Geometry check sheet. Reference: the model listing, model coordinates, mm. Face numbers are marked on the shaded views. Round coordinates to 2 decimals unless told otherwise and drop trailing zeros. Loops run counter-clockwise (first coordinate to the right, second up) from the corner with the lowest first, then second, coordinate; pieces in that order, holes last. Notation, with made-up numbers: M -10,82.5 L 5,82.5 A29 cw 5,113.5 Z; hole C 72.5,-19.75 d4. An arc over 180 degrees is marked long. Answer in a Markdown table with one row per item. Add a question column.
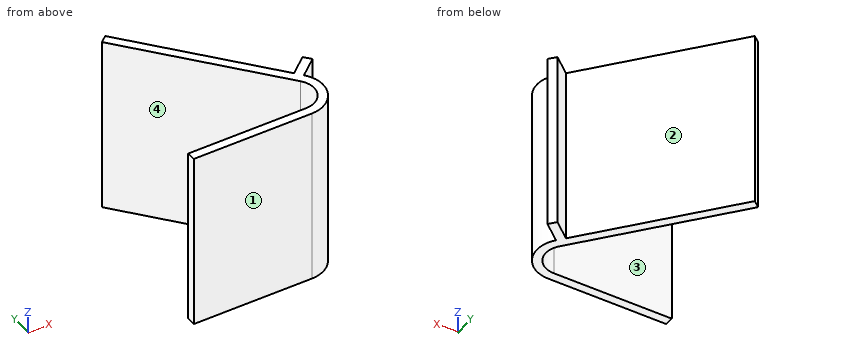
```python
from build123d import *

# Parameters (mm, degrees)
F1_DEPTH = 152.4


with BuildPart() as f1:
    # F0 (on Top) → F1 (new body)
    with BuildSketch(Plane.XY):
        with BuildLine():
            Line((-114.31821, -32.882527), (-114.198142, -40.501581))
            Line((-114.198142, -40.501581), (-12.598142, -40.501581))
            ThreePointArc((-12.598142, -40.501581), (10.422075, -25.836085), (6.859386, 1.225224))
            Line((6.859386, 1.225224), (22.425409, 14.286668))
            Line((22.425409, 14.286668), (17.527368, 20.123927))
            Line((17.527368, 20.123927), (1.961345, 7.062483))
            Line((1.961345, 7.062483), (-91.101445, 117.970397))
            Line((-91.101445, 117.970397), (-96.938704, 113.072356))
            Line((-96.938704, 113.072356), (1.022921, -3.673763))
            ThreePointArc((1.022921, -3.673763), (3.516804, -22.61668), (-12.597349, -32.882527))
            Line((-12.597349, -32.882527), (-114.31821, -32.882527))
        make_face()
    extrude(amount=F1_DEPTH)


solid = f1.part
```
1) Cross-section at A-A, the plane z = 85. Record the boundary of the cut face in (x, y), plus the area to 3 significant figures.
2) Cross-section at C-C, the plane x = -100.5. Record the boundary of the cut face in (y, z).
3) Thickness scan on L1, parallel to Y at x = -106, z = 68.5; L2, parallel to Y at x = -76, z = 143; L3, parallel to X at y = 14, z = 54.5. Record the ranges inside material, lowest first. Write a range as [from, to].
4) Cross-section at D-D, the plane y = 106. Record the boundary of the cut face in (x, z).
5) Go/stop test with flat-tipped pins: pin 1 (10 mm diameter, centred on x = -95.5, z = 124, fed in from +Y); pin 2 (6 mm diameter, centred on y = 18.5, z = 38.5, fed in from -X); pin 3 (12 mm diameter, centred on x = -4.5, z = 84, fed in from +Y). Record where each tip stops, or that it passes through.
6) Draft check along Y on the marked faces 1, 2, 3 and 4. Enter one of: +Y half, -Y half, draft (parallel to the pull), parting line (faces both ways), or undercut.
7) Cross-section at B-B, the plane x = -18. Record the boundary of the cut face in (y, z), plus the area to 3 significant figures.
Worked answers:
| question | item | result |
|---|---|---|
| 1 | outline | M -114.32,-32.88 L -114.2,-40.5 L -12.6,-40.5 A25.4 ccw 6.86,1.23 L 22.43,14.29 L 17.53,20.12 L 1.96,7.06 L -91.1,117.97 L -96.94,113.07 L 1.02,-3.67 A17.78 cw -12.6,-32.88 Z |
| 1 | area | 2,460 mm2 |
| 2 | outline | M -40.5,0 L -32.88,0 L -32.88,152.4 L -40.5,152.4 Z |
| 3 | L1 | y = [-40.5, -32.88] |
| 3 | L2 | y = [-40.5, -32.88], [88.12, 99.97] |
| 3 | L3 | x = [-13.81, -3.86], [10.23, 22.08] |
| 4 | outline | M -91,0 L -81.06,0 L -81.06,152.4 L -91,152.4 Z |
| 5 | pin 1 | stops at y = 117.97 |
| 5 | pin 2 | stops at x = -20.1 |
| 5 | pin 3 | stops at y = 21.91 |
| 6 | face 1 | -Y half |
| 6 | face 2 | +Y half |
| 6 | face 3 | undercut |
| 6 | face 4 | undercut |
| 7 | outline | M -40.5,0 L -32.88,0 L -32.88,152.4 L -40.5,152.4 Z; M 19,0 L 30.85,0 L 30.85,152.4 L 19,152.4 Z |
| 7 | area | 2,970 mm2 |
